```python
from build123d import *

# Parameters (mm, degrees)
SKETCH_R     = 30
PAD_DEPTH    = 30
SKETCH001_R  = 35
PAD001_DEPTH = 40
SKETCH002_R  = 37.5
POCKET_DEPTH = 35
PAD002_DEPTH = 10


with BuildPart() as part:
    # Sketch → Pad (new body)
    with BuildSketch(Plane.XY):
        Circle(SKETCH_R)
    extrude(amount=PAD_DEPTH)

    # Sketch001 → Pad001 (join)
    with BuildSketch(Plane.YZ):
        with Locations((0, 35)):
            Circle(SKETCH001_R)
    extrude(amount=-PAD001_DEPTH)

    # Sketch002 → Pocket (cut)
    with BuildSketch(Plane.YZ):
        with Locations((0, 35)):
            Circle(SKETCH002_R)
    extrude(amount=POCKET_DEPTH, mode=Mode.SUBTRACT)

    # Sketch → Pad002 (join)
    with BuildSketch(Plane.XY):
        Circle(SKETCH_R)
    extrude(amount=-PAD002_DEPTH)


solid = part.part
```
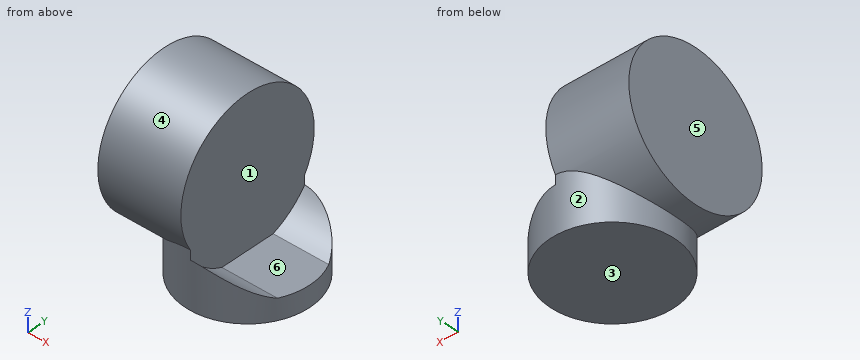
Design review of the part built by this model. Coordinates are the model's own, in mm. Face numbers are marked on the shaded views. A direction names the side the tool comes from. Coordinates: 2 decimals unless noted, no trailing zeros. Order: outer loops, then holes, each group sorted by start corner. A loop starts at its lowest first (then second) coordinate and runs counter-clockwise, first axis right, second up.
1) For the marked faces 1, 2 and 3, list the 3-axis set-ups (+Z, -Z, +X, -X, +Y, -Y) from which the entire face can be reached by the end or side of a thin tool; tool diameter is ignored.
2) Mouldability with a two-part tool opening along Y and no side actions: class the marked faces 4, 5 and 6 as +Y half, -Y half, draft (parallel to the pull), parting line (faces both ways), or undercut.
3) Take a section at B-B, the plane x = 19.5. Give the boundary of the cut face in (y, z).
4) Wall thickness on line 1 along X through (y, z) = (27.5, 29.5); line 2 along Y through (x, z) = (-28.5, 37); line 3 along Y through (x, z) = (-24, 19): over which ranges is each line inside the solid? List them lowest first.
5) Clearance check with flat-ended pins moving along their axes: pin 1 (21 mm diameter, centred on y = 2, z = 52.5, fed in from +X); pin 2 (21.5 mm diameter, centred on x = 19, y = -5, fed in from +Z); pin 3 (8 mm diameter, centred on x = -17, z = 19, fed in from -Y). State where each tip first meets the part, or that it passes through.
6) Take a section at C-C, the plane z = 35. Give the boundary of the cut face in (x, y), and give its area (3 significant figures).
7) Take a section at A-A, the plane y = 0. Give the boundary of the cut face in (x, z), and give its area (3 significant figures).
8) Take a section at D-D, the plane y = -15.5. Give the boundary of the cut face in (x, z), and give its area (3 significant figures).
Returned:
1. face 1: +Z, +X
1. face 2: -Z
1. face 3: -Z, +X, -X, +Y, -Y
2. face 4: parting line
2. face 5: draft
2. face 6: undercut
3. outline: (-22.8, -10) - (22.8, -10) - (22.8, 5.23) arc R37.5 cw to (13.46, 0) - (-13.46, 0) arc R37.5 cw to (-22.8, 5.23) - close
4. line 1: x = -40 to 0
4. line 2: y = -34.94 to 34.94
4. line 3: y = -31.13 to 31.13
5. pin 1: stops at x = 0
5. pin 2: stops at z = 0.97
5. pin 3: stops at y = -32.88
6. outline: (-40, -35) - (0, -35) - (0, 35) - (-40, 35) - close
6. area: 2,800 mm2
7. outline: (-40, 0) - (-30, 0) - (-30, -10) - (30, -10) - (30, 0) - (0, 0) - (0, 70) - (-40, 70) - close
7. area: 3,400 mm2
8. outline: (-40, 3.62) - (-25.69, 3.62) - (-25.69, -10) - (25.69, -10) - (25.69, 0.85) - (0, 0.85) - (0, 66.38) - (-40, 66.38) - close
8. area: 3,140 mm2
